from build123d import *

# Parameters (mm, degrees)
BOSS_EXTRUDE1_DEPTH     = 25.4
SKETCH2_W               = 15.4
SKETCH2_H               = 20.48
CUT_EXTRUDE1_DEPTH      = 25.4
CUT_EXTRUDE2_DEPTH      = 48.109981957
CUT_EXTRUDE2_DEPTH_BACK = 48.109981957
CUT_EXTRUDE3_DEPTH      = 48.153163202
CUT_EXTRUDE3_DEPTH_BACK = 48.153163202


with BuildPart() as part:
    # Sketch1 → Boss-Extrude1 (new body)
    with BuildSketch(Plane(origin=(0, 0, 0), x_dir=(0, 0, -1), z_dir=(1, 0, 0))):
        Polygon((0, 0), (30.48, 0), (30.48, 30.48), (25.48, 30.48), (25.48, 25.48), (5, 5), (0, 5), align=None)
    extrude(amount=BOSS_EXTRUDE1_DEPTH)

    # Sketch2 → Cut-Extrude1 (cut)
    with BuildSketch(Plane.XY):
        with Locations((12.7, 15.24)):
            Rectangle(SKETCH2_W, SKETCH2_H)
    extrude(amount=-CUT_EXTRUDE1_DEPTH, mode=Mode.SUBTRACT)

    # Sketch3 → Cut-Extrude2 (cut, two sides: drawn at the far end of the back side and taken through both)
    with BuildSketch(Plane.XY.offset(-25.4).offset(-CUT_EXTRUDE2_DEPTH_BACK)):
        with BuildLine():
            Line((15.7, 18.2), (15.7, 12.2))
            ThreePointArc((15.7, 12.2), (12.7, 9.2), (9.7, 12.2))
            Line((9.7, 12.2), (9.7, 18.2))
            ThreePointArc((9.7, 18.2), (12.7, 21.2), (15.7, 18.2))
        make_face()
    extrude(amount=CUT_EXTRUDE2_DEPTH + CUT_EXTRUDE2_DEPTH_BACK, mode=Mode.SUBTRACT)

    # Sketch4 → Cut-Extrude3 (cut, two sides: drawn at the far end of the back side and taken through both)
    with BuildSketch(Plane(origin=(0, 5, 0), x_dir=(1, 0, 0), z_dir=(0, 1, 0)).offset(-CUT_EXTRUDE3_DEPTH_BACK)):
        with BuildLine():
            Line((15.7, 18.2), (15.7, 12.2))
            ThreePointArc((15.7, 12.2), (12.7, 9.2), (9.7, 12.2))
            Line((9.7, 12.2), (9.7, 18.2))
            ThreePointArc((9.7, 18.2), (12.7, 21.2), (15.7, 18.2))
        make_face()
    extrude(amount=CUT_EXTRUDE3_DEPTH + CUT_EXTRUDE3_DEPTH_BACK, mode=Mode.SUBTRACT)


solid = part.part
The listing builds one solid part. Answer for the finished solid, in the listing's coordinates (mm). A direction names the side the tool comes from. Round coordinates to 2 decimals unless told otherwise and drop trailing zeros. Order: outer loops, then holes, each group sorted by start corner. A loop starts at its lowest first (then second) coordinate and runs counter-clockwise, first axis right, second up. Notation, with made-up numbers: (31, 6.5) -> (70, 6.5) arc R7 ccw to (70, 15.5) -> close; hole circle Ø5 at (3.5, 35.25). An arc over 180 degrees is marked (long way). Write each question's results on one line, items separated by ' | '. Start each with the question number.
Q1. Find section A-A (x = 12.7). Determine the outline of the cut face in (y, z), then the cut area to 3 significant figures.
Q2. Straight lines are drawn through the part: probe 1 along X at (y, z) = (8, -8.5); probe 2 along Y at (x, z) = (13.5, -7.5); probe 3 along Z at (x, y) = (19.25, 10). For each, find the intervals that lie inside material, in ascending order. Write a range as from..to.
Q3. Find section B-B (z = -28). Determine the outline of the cut face in (x, y).
Q4. Each of these flat-tipped pins is pushed along its axis until it touches: pin 1 (8 mm diameter, centred on x = 13, y = 13, fed in from +Z); pin 2 (1.5 mm diameter, centred on x = 13, y = 27.5, fed in from +Z); pin 3 (1 mm diameter, centred on x = 19.5, z = -9, fed in from +Y). Where does it stop, or does it pass through?
Q5. The mould has two halves that part along Y. Classify faces 1 (the cylindrical face through (12.8, 9.2, -28)), 2 (the flat face through (13, 3, 0)), 3 (the flat face through (13, 30.48, -28)): pulls with the +Y half, pulls with the -Y half, needs draft (parallel to the pull), parting line crosses it, or undercut.
Q6. Find section D-D (z = -11.5). Determine the outline of the cut face in (x, y).
Q7. Find section C-C (y = 4.5). Determine the outline of the cut face in (x, z).
Q8. Which of the six approach directions +Z, -Z, +X, -X, +Y, -Y give full straight-line access (tool end or side, diameter ignored) to faces 4 (the flat face through (15.7, 2, -15)), 5 (the flat face through (16, 15, -25.4)), 6 (the cylindrical face through (12.6, 21.2, -28))?
Worked answers:
1) outline: (0, -30.48) -> (9.2, -30.48) -> (9.2, -25.4) -> (5, -25.4) -> (5, -21.2) -> (0, -21.2) -> close; (0, -9.2) -> (5, -9.2) -> (5, 0) -> (0, 0) -> close; (21.2, -30.48) -> (30.48, -30.48) -> (30.48, -25.48) -> (25.48, -25.48) -> (25.4, -25.4) -> (21.2, -25.4) -> close | area: 160 mm2
2) probe 1: x = 0..5, 20.4..25.4 | probe 2: y = 0..5 | probe 3: z = -30.48..-25.4
3) outline: (0, 0) -> (25.4, 0) -> (25.4, 30.48) -> (0, 30.48) -> close; hole (9.7, 12.2) arc R3 ccw to (15.7, 12.2) -> (15.7, 18.2) arc R3 ccw to (9.7, 18.2) -> close
4) pin 1: stops at z = -25.4 | pin 2: stops at z = -25.48 | pin 3: stops at y = 5
5) face 1: undercut | face 2: needs draft | face 3: pulls with the +Y half
6) outline: (0, 0) -> (9.78, 0) -> (9.78, 5) -> (5, 5) -> (5, 11.5) -> (0, 11.5) -> close; (15.62, 0) -> (25.4, 0) -> (25.4, 11.5) -> (20.4, 11.5) -> (20.4, 5) -> (15.62, 5) -> close
7) outline: (0, -30.48) -> (25.4, -30.48) -> (25.4, 0) -> (0, 0) -> close; hole (9.7, -18.2) arc R3 ccw to (15.7, -18.2) -> (15.7, -12.2) arc R3 ccw to (9.7, -12.2) -> close
8) face 4: +Y, -Y | face 5: +Z, +Y | face 6: +Z, -Z
